Design review of the part shown in the three views and the two pictorial views. Dimensions are in mm from the part's minimum x, y and z. Round coordinates to 2 decimals unless told otherwise and drop trailing zeros. Order: outer loops, then holes, each group sorted by start corner. A loop starts at its lowest first (then second) coordinate and runs counter-clockwise, first axis right, second up. Notation, with made-up numbers: M 20.5,-36.5 L 71.5,-36.5 A33 ccw 71.5,-2.5 Z; hole C 22.5,-30.75 d9. An arc over 180 degrees is marked long. Use a Markdown table: item, result. Add a question column.
(1) Take a section at C-C (z = 3.75). Write out the cut boundary in (x, y).
(2) To check wall thickness, follow probe 1 along Y at (x, z) = (7.5, 6.65); probe 2 along Y at (x, z) = (12, 7.5). State the ranges of each line that lie inside material, in increasing order. Write a range as from..to.
(3) Take a section at D-D (z = 1.25). Write out the cut boundary in (x, y).
(4) The part is to be moulded in two halves that separate along Z. For the marked faces 1, 2 and 3, say which applies: released by +Z, released by -Z, zero draft, split by the parting line, or undercut.
(5) For pin 1 (1.5 mm diameter, centred on x = 13.5, z = 4.5, fed in from +Y); pin 2 (1.5 mm diameter, centred on x = 9.5, z = 5.5, fed in from +Y); pin 3 (5 mm diameter, centred on y = 4, z = 8, fed in from +X); pin 4 (9 mm diameter, centred on x = 7.5, y = 7.5, fed in from +Z), all flat-tipped, find the tip position at first contact; note any pin that passes through.
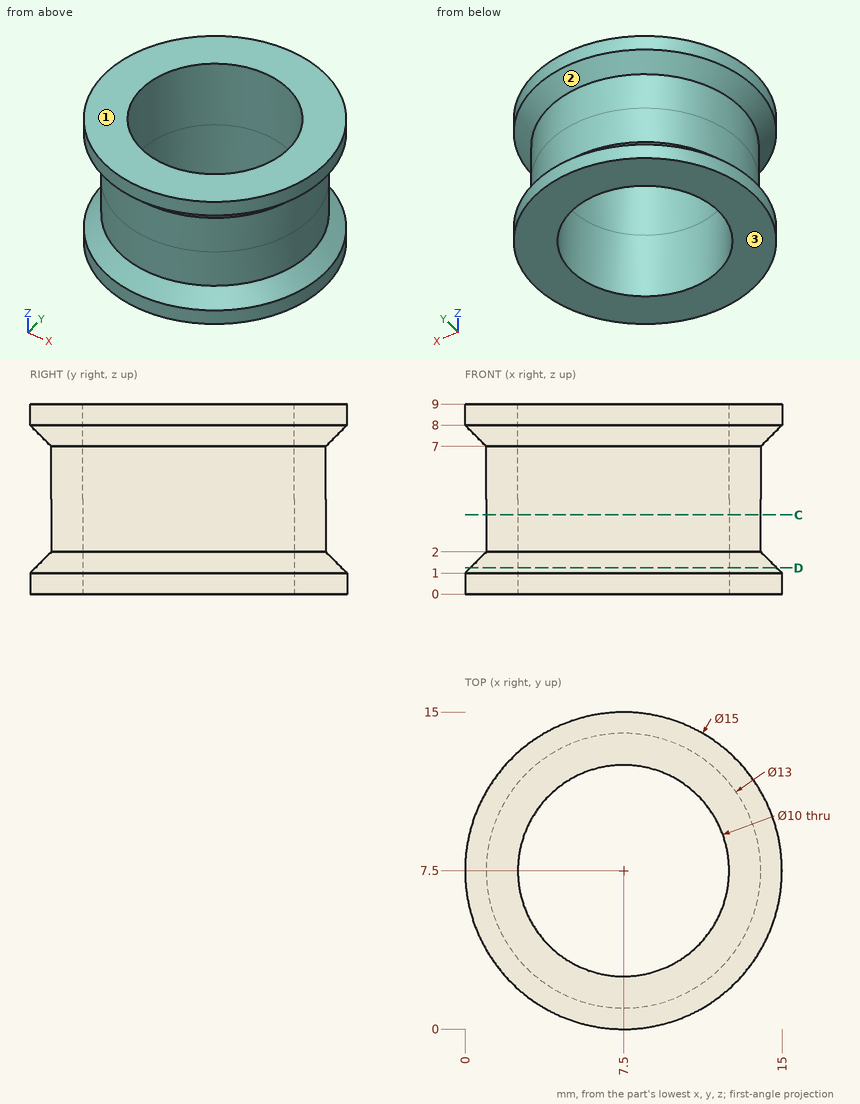
Verdict:
| question | item | result |
|---|---|---|
| 1 | outline | C 7.5,7.5 d13; hole C 7.5,7.5 d10 |
| 2 | probe 1 | y = 1..2.5, 12.5..14 |
| 2 | probe 2 | y = 2.14..5.32, 9.68..12.86 |
| 3 | outline | C 7.5,7.5 d14.5; hole C 7.5,7.5 d10 |
| 4 | face 1 | released by +Z |
| 4 | face 2 | undercut |
| 4 | face 3 | released by -Z |
| 5 | pin 1 | stops at y = 11.33 |
| 5 | pin 2 | stops at y = 13.88 |
| 5 | pin 3 | stops at x = 14.93 |
| 5 | pin 4 | passes through |
